Part model, mm, in its own coordinate system. A direction names the side the tool comes from. Round coordinates to 2 decimals unless told otherwise and drop trailing zeros. Write each loop counter-clockwise with the first axis right and the second up, starting at its lowest first coordinate (ties: lowest second). Pieces come first, ordered by that corner, then holes.
1) Saw through at B-B on z = 4. Count the separate pieces of the cut face and the enclosed holes in it, and give its area (3 significant figures).
2) Pull direction Z, two halves, no side cores. Call faces 1 (the cylindrical face through (-22.67, 18.2, 2.54)), 2 (the flat face through (-47.403, 12, 9)): +Z half, -Z half, draft (parallel to the pull), parting line (faces both ways), or undercut.
3) Saw through at A-A on x = -43. Write the cut outline in (y, z).
4) Which spindle directions (+Z, -Z, +X, -X, +Y, -Y) get a long thin tool onto all of the face, cutting with end or side? Do faces 3 (the flat face through (-80.403, 30, 3)), 4 (the cylindrical face through (19.83, 18.2, 2.54)), 5 (the flat face through (9.597, 12, 9)), 6 (the flat face through (26.597, 18, 1)). Say none if no direction does.
5) Flat gauge pins, fed straight in: pin 1 (17 mm diameter, centred on x = 13, y = 28, fed in from +Z); pin 2 (6.5 mm diameter, centred on x = -68.5, y = 29.5, fed in from +Z); pin 3 (2.5 mm diameter, centred on x = -35.9, y = 19.18, fed in from -Z) (3 decimals). Where does each tip first touch, or does it go through?
6) Drill centre lines: L1, parallel to X at y = 35, z = 10.75; L2, parallel to X at y = 36, z = 4.5; L3, parallel to Y at x = -38.5, z = 13.25. Where is each one in solid material? Low to high.
```python
from build123d import *

# Parameters (mm, degrees)
SKETCH_1_W          = 114
SKETCH_1_H          = 30
EXTRUDE_1_DEPTH     = 15
SKETCH_2_W          = 21
SKETCH_2_H          = 26
CUT_EXTRUDE_1_DEPTH = 13
SKETCH_3_W          = 21
SKETCH_3_H          = 26
SKETCH_3_W_2        = 18
SKETCH_3_H_2        = 23
EXTRUDE_2_DEPTH     = 3
SKETCH_5_W          = 4.5
SKETCH_5_H          = 6
EXTRUDE_3_DEPTH     = 3
SKETCH_6_R          = 1.6
CUT_EXTRUDE_2_DEPTH = 94.778887913
SKETCH_7_W          = 9
SKETCH_7_H          = 8
CUT_EXTRUDE_3_DEPTH = 90.714734825
SKETCH_12_W         = 2
SKETCH_12_H         = 5
CUT_EXTRUDE_4_DEPTH = 3.5


with BuildPart() as part:
    # ｽｹｯﾁ1 → ﾎﾞｽ - 押し出し1 (new body)
    with BuildSketch(Plane.XY):
        with Locations((-26.90312059, 25.678571429)):
            Rectangle(SKETCH_1_W, SKETCH_1_H)
    extrude(amount=EXTRUDE_1_DEPTH)

    # ｽｹｯﾁ2 → ｶｯﾄ - 押し出し1 (cut)
    with BuildSketch(Plane.XY.offset(15)):
        with Locations((-71.40312059, 25.678571429)):
            Rectangle(SKETCH_2_W, SKETCH_2_H)
        with Locations((-42.90312059, 25.678571429)):
            Rectangle(SKETCH_2_W, SKETCH_2_H)
        with Locations((-14.40312059, 25.678571429)):
            Rectangle(SKETCH_2_W, SKETCH_2_H)
        with Locations((14.09687941, 25.678571429)):
            Rectangle(SKETCH_2_W, SKETCH_2_H)
    extrude(amount=-CUT_EXTRUDE_1_DEPTH, mode=Mode.SUBTRACT)

    # ｽｹｯﾁ3 → ﾎﾞｽ - 押し出し2 (add)
    # profile 1 of 4: a face of its own
    with BuildSketch(Plane.XY.offset(2)):
        with Locations((-71.40312059, 25.678571429)):
            Rectangle(SKETCH_3_W, SKETCH_3_H)
        with Locations((-71.40312059, 25.678571429)):
            Rectangle(SKETCH_3_W_2, SKETCH_3_H_2, mode=Mode.SUBTRACT)
    # profile 2 of 4: a face of its own
    with BuildSketch(Plane.XY.offset(2)):
        with Locations((-42.90312059, 25.678571429)):
            Rectangle(SKETCH_3_W, SKETCH_3_H)
        with Locations((-42.90312059, 25.678571429)):
            Rectangle(SKETCH_3_W_2, SKETCH_3_H_2, mode=Mode.SUBTRACT)
    # profile 3 of 4: a face of its own
    with BuildSketch(Plane.XY.offset(2)):
        with Locations((-14.40312059, 25.678571429)):
            Rectangle(SKETCH_3_W, SKETCH_3_H)
        with Locations((-14.40312059, 25.678571429)):
            Rectangle(SKETCH_3_W_2, SKETCH_3_H_2, mode=Mode.SUBTRACT)
    # profile 4 of 4: a face of its own
    with BuildSketch(Plane.XY.offset(2)):
        with Locations((14.09687941, 25.678571429)):
            Rectangle(SKETCH_3_W, SKETCH_3_H)
        with Locations((14.09687941, 25.678571429)):
            Rectangle(SKETCH_3_W_2, SKETCH_3_H_2, mode=Mode.SUBTRACT)
    extrude(amount=EXTRUDE_2_DEPTH)

    # ｽｹｯﾁ5 → ﾎﾞｽ - 押し出し3 (add)
    with BuildSketch(Plane.XY.offset(2)):
        with Locations((-64.65312059, 19.178571429)):
            Rectangle(SKETCH_5_W, SKETCH_5_H)
        with Locations((-78.15312059, 19.178571429)):
            Rectangle(SKETCH_5_W, SKETCH_5_H)
        with Locations((-49.65312059, 19.178571429)):
            Rectangle(SKETCH_5_W, SKETCH_5_H)
        with Locations((-36.15312059, 19.178571429)):
            Rectangle(SKETCH_5_W, SKETCH_5_H)
        with Locations((-21.15312059, 19.178571429)):
            Rectangle(SKETCH_5_W, SKETCH_5_H)
        with Locations((-7.65312059, 19.178571429)):
            Rectangle(SKETCH_5_W, SKETCH_5_H)
        with Locations((7.34687941, 19.178571429)):
            Rectangle(SKETCH_5_W, SKETCH_5_H)
        with Locations((20.84687941, 19.178571429)):
            Rectangle(SKETCH_5_W, SKETCH_5_H)
    extrude(amount=EXTRUDE_3_DEPTH)

    # ｽｹｯﾁ6 → ｶｯﾄ - 押し出し2 (cut, through all)
    with BuildSketch(Plane.XY.offset(5)):
        with Locations((-64.40312059, 19.178571429)):
            Circle(SKETCH_6_R)
        with Locations((-78.40312059, 19.178571429)):
            Circle(SKETCH_6_R)
        with Locations((-49.90312059, 19.178571429)):
            Circle(SKETCH_6_R)
        with Locations((-35.90312059, 19.178571429)):
            Circle(SKETCH_6_R)
        with Locations((-21.40312059, 19.178571429)):
            Circle(SKETCH_6_R)
        with Locations((-7.40312059, 19.178571429)):
            Circle(SKETCH_6_R)
        with Locations((7.09687941, 19.178571429)):
            Circle(SKETCH_6_R)
        with Locations((21.09687941, 19.178571429)):
            Circle(SKETCH_6_R)
    extrude(amount=-CUT_EXTRUDE_2_DEPTH, mode=Mode.SUBTRACT)

    # ｽｹｯﾁ7 → ｶｯﾄ - 押し出し3 (cut, through all)
    with BuildSketch(Plane(origin=(0, 12.678571429, 0), x_dir=(1, 0, 0), z_dir=(0, 1, 0))):
        with Locations((-71.40312059, -9)):
            Rectangle(SKETCH_7_W, SKETCH_7_H)
        with Locations((-42.90312059, -9)):
            Rectangle(SKETCH_7_W, SKETCH_7_H)
        with Locations((-14.40312059, -9)):
            Rectangle(SKETCH_7_W, SKETCH_7_H)
        with Locations((14.09687941, -9)):
            Rectangle(SKETCH_7_W, SKETCH_7_H)
    extrude(amount=-CUT_EXTRUDE_3_DEPTH, mode=Mode.SUBTRACT)

    # ｽｹｯﾁ12 → ｶｯﾄ - 押し出し4 (cut)
    with BuildSketch(Plane(origin=(30.09687941, 0, 0), x_dir=(0, 0, -1), z_dir=(1, 0, 0))):
        with Locations((-1, 18.178571429)):
            Rectangle(SKETCH_12_W, SKETCH_12_H)
        with Locations((-1, 33.178571429)):
            Rectangle(SKETCH_12_W, SKETCH_12_H)
    extrude(amount=-CUT_EXTRUDE_4_DEPTH, mode=Mode.SUBTRACT)


solid = part.part
```
Completed:
1. separate pieces: 1
1. enclosed holes: 12
1. area: 1,920 mm2
2. face 1: draft
2. face 2: undercut
3. outline: (10.68, 0) - (40.68, 0) - (40.68, 15) - (38.68, 15) - (38.68, 5) - (37.18, 5) - (37.18, 2) - (14.18, 2) - (14.18, 5) - (10.68, 5) - close; (10.68, 13) - (12.68, 13) - (12.68, 15) - (10.68, 15) - close
4. face 3: +Z
4. face 4: +Z, -Z
4. face 5: -Y
4. face 6: -Z, +X
5. pin 1: stops at z = 5
5. pin 2: stops at z = 2
5. pin 3: passes through
6. L1: x = -83.9 to -81.9, -60.9 to -53.4, -32.4 to -24.9, -3.9 to 3.6, 24.6 to 30.1
6. L2: x = -83.9 to -80.4, -62.4 to -51.9, -33.9 to -23.4, -5.4 to 5.1, 23.1 to 30.1
6. L3: y = 10.68 to 12.68, 38.68 to 40.68
